The model under review builds one solid part; all positions refer to its coordinate system, in mm. Round coordinates to 2 decimals unless told otherwise and drop trailing zeros. Write each loop counter-clockwise with the first axis right and the second up, starting at its lowest first coordinate (ties: lowest second). Pieces come first, ordered by that corner, then holes. Notation, with made-up numbers: (-11, 89.25) -> (24, 89.25) arc R23 cw to (24, 114.25) -> close; hole circle Ø9 at (83, -5). An arc over 180 degrees is marked (long way). Use CSV: the item, a comma, the result in double quotes. Start each with the question number.
1) Take a section at B-B, the plane x = -28. Give the boundary of the cut face in (y, z), then the cut area to 4 significant figures.
2) For pin 1 Ø1.5 at (x, y) = (-22, 1.5) entering from +Z; pin 2 Ø0.9 at (y, z) = (1, -15.5) entering from -X; pin 3 Ø0.9 at (x, y) = (-24.5, 2) entering from -Z, all flat-tipped, find the tip position at first contact; note any pin that passes through.
3) Wall thickness on probe 1 along Z at (x, y) = (-13, 2.35); probe 2 along X at (y, z) = (2.7, -141): over which ranges is each line inside the solid? List them lowest first. Write a range as [from, to].
4) Take a section at A-A, the plane y = 2.25. Give the boundary of the cut face in (x, z).
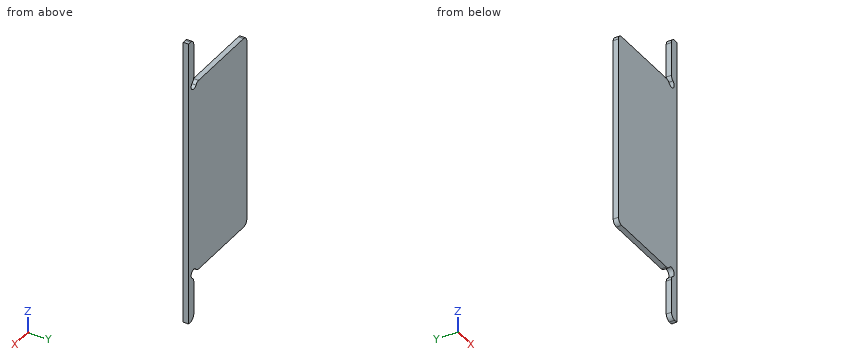
Autodesk Inventor part; units mm, degrees
ref_plane "YZ Plane" through (0, 0, 0) normal (1, 0, 0) x (0, 1, 0)
ref_plane "XZ Plane" through (0, 0, 0) normal (0, 1, 0) x (-1, 0, 0)
ref_plane "XY Plane" through (0, 0, 0) normal (0, 0, 1) x (1, 0, 0)
sketch "Sketch1" plane through (0, 0, 0) normal (0, 1, 0) x (-1, 0, 0)
  line L0 (55, -30) -> (55, -135.5)
  line L1 (0, -165.5) -> (0, 0)
  line L2 (52, -27) -> (9.6098, -27)
  line L3 (0, -27) -> (0, 0)
  line L4 (52, -138.5) -> (9.6098, -138.5)
  line L5 (0, -138.5) -> (0, -165.5)
  line L6 (0, 0) -> (2, 0)
  line L7 (5, -3) -> (5, -22.3902)
  line L8 (0, -27) -> (0, 0)
  line L9 (0, -165.5) -> (2, -165.5)
  line L10 (5, -162.5) -> (5, -143.1098)
  line L11 (0, -138.5) -> (0, -165.5)
  arc A0 (3.6364, -24.9046) -> (7.0954, -28.3636) centre (5, -27) ccw
  arc A1 (7.0954, -137.1364) -> (3.6364, -140.5954) centre (5, -138.5) ccw
  arc A2 (55, -30) -> (52, -27) centre (52, -30) ccw
  arc A3 (52, -138.5) -> (55, -135.5) centre (52, -135.5) ccw
  arc A4 (9.6098, -27) -> (7.0954, -28.3636) centre (9.6098, -30) ccw
  arc A5 (3.6364, -24.9046) -> (5, -22.3902) centre (2, -22.3902) ccw
  arc A6 (7.0954, -137.1364) -> (9.6098, -138.5) centre (9.6098, -135.5) ccw
  arc A7 (5, -143.1098) -> (3.6364, -140.5954) centre (2, -143.1098) ccw
  arc A8 (5, -3) -> (2, 0) centre (2, -3) ccw
  arc A9 (2, -165.5) -> (5, -162.5) centre (2, -162.5) ccw
  point P0 (5, -24.5)
  point P1 (5, -141)
  point P2 (7.5, -27)
  point P3 (7.5, -138.5)
  dimension "d8" = 3
  dimension "d9" = 3
extrude "Extrusion1" add sketch "Sketch1" along normal blind 3
properties part number "Maze Wall Alignment Jig"
Values found:
1,outline,"(0, -138.5) -> (3, -138.5) -> (3, -27) -> (0, -27) -> close"
1,area,"334.5 mm²"
2,pin 1,"z = -27"
2,pin 2,"x = -5"
2,pin 3,"z = -138.5"
3,probe 1,"[-138.5, -27]"
3,probe 2,"[-4.13, 0]"
4,outline,"(-55, -135.5) arc R3 ccw to (-52, -138.5) -> (-9.61, -138.5) arc R3 ccw to (-7.1, -137.14) arc R2.5 cw (long way) to (-3.64, -140.6) arc R3 ccw to (-5, -143.11) -> (-5, -162.5) arc R3 ccw to (-2, -165.5) -> (0, -165.5) -> (0, 0) -> (-2, 0) arc R3 ccw to (-5, -3) -> (-5, -22.39) arc R3 ccw to (-3.64, -24.9) arc R2.5 cw (long way) to (-7.1, -28.36) arc R3 ccw to (-9.61, -27) -> (-52, -27) arc R3 ccw to (-55, -30) -> close"
